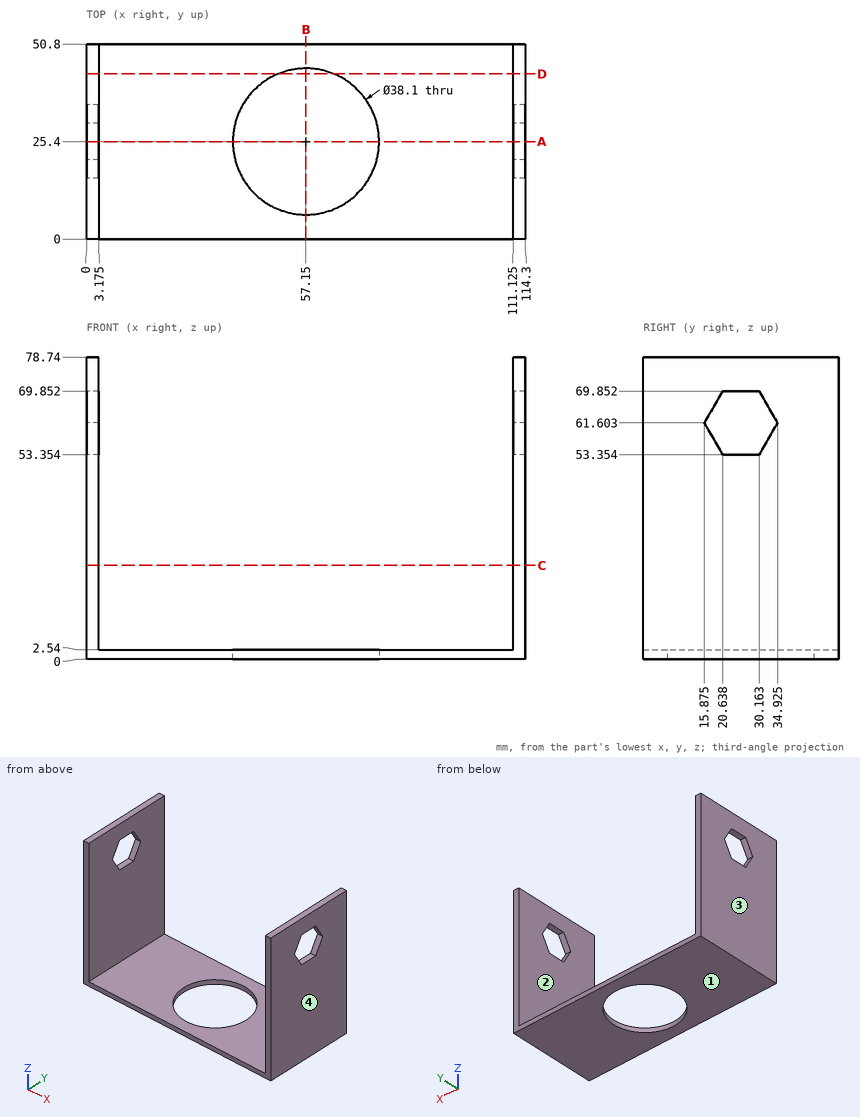
Study the drawing (mm; zero at the part's minimum x, y, z) and answer. Give positions to 0.01 mm unless a question says otherwise; leave off trailing zeros. Write each loop counter-clockwise with the first axis right and the second up, starting at its lowest first coordinate (ties: lowest second). Pieces come first, ordered by that corner, then holes. Notation, with made-up numbers: (35.5, 37) - (78.5, 37) arc R35 ccw to (78.5, 72) - close; hole circle Ø7 at (24.25, 65). An arc over 180 degrees is marked (long way). Use CSV: the item, a comma, the result in double quotes. Start each with the question number.
(1) Find section A-A (y = 25.4). Give the vertices of the cut face in (x, z) (1 decimal).
(2) Consider line 1 along Y through (x, z) = (57, 1); line 2 along X through (y, z) = (43.5, 22.5) (1 decimal); line 3 along X through (y, z) = (25, 1) (1 decimal). Determine where each line is inside the solid, lowest interval first.
(3) Find section D-D (y = 43). Give the vertices of the cut face in (x, z) (1 decimal).
(4) Find section B-B (x = 57.15). Give the vertices of the cut face in (y, z).
(5) Determine the mould class of the marked faces 1, 2, 3 and 4 for opening direction X: +X half, -X half, draft (parallel to the pull), parting line (faces both ways), or undercut.
(6) Find section C-C (z = 24.5). Give the vertices of the cut face in (x, y) (1 decimal).
(7) Given P1, Ø3, axis at x = 40.5, y = 23, coming from the -Z side; P2, Ø1.5, axis at x = 17.5, y = 18.5, coming from the +Z side, each flat-ended and moving along its own axis, determine where each tip first touches the part or whether it passes through.
Findings below:
1,outline,"(0, 0) - (38.1, 0) - (38.1, 2.5) - (3.2, 2.5) - (3.2, 53.4) - (0, 53.4) - close; (0, 69.9) - (3.2, 69.9) - (3.2, 78.7) - (0, 78.7) - close; (76.2, 0) - (114.3, 0) - (114.3, 53.4) - (111.1, 53.4) - (111.1, 2.5) - (76.2, 2.5) - close; (111.1, 69.9) - (114.3, 69.9) - (114.3, 78.7) - (111.1, 78.7) - close"
2,line 1,"0 to 6.35, 44.45 to 50.8"
2,line 2,"0 to 3.2, 111.1 to 114.3"
2,line 3,"0 to 38.1, 76.2 to 114.3"
3,outline,"(0, 0) - (49.9, 0) - (49.9, 2.5) - (3.2, 2.5) - (3.2, 78.7) - (0, 78.7) - close; (64.4, 0) - (114.3, 0) - (114.3, 78.7) - (111.1, 78.7) - (111.1, 2.5) - (64.4, 2.5) - close"
4,outline,"(0, 0) - (6.35, 0) - (6.35, 2.54) - (0, 2.54) - close; (44.45, 0) - (50.8, 0) - (50.8, 2.54) - (44.45, 2.54) - close"
5,face 1,"draft"
5,face 2,"undercut"
5,face 3,"-X half"
5,face 4,"+X half"
6,outline,"(0, 0) - (3.2, 0) - (3.2, 50.8) - (0, 50.8) - close; (111.1, 0) - (114.3, 0) - (114.3, 50.8) - (111.1, 50.8) - close"
7,P1,"through"
7,P2,"z = 2.54"
